Read the model definition and answer for the solid it produces. Units are mm, in the model's axes. Give positions to 0.01 mm unless a question says otherwise; leave off trailing zeros. Order: outer loops, then holes, each group sorted by start corner. A loop starts at its lowest first (then second) coordinate and runs counter-clockwise, first axis right, second up.
Item 1: A cutting plane is placed at B-B (z = 0.7). State how many separate pieces and enclosed holes the cut face has, plus the area to 3 significant figures.
Item 2: A cutting plane is placed at A-A (x = -188). Write down the section's boundary in (y, z), plus the area to 3 significant figures.
Item 3: Given pin 1 Ø3.5 at (x, y) = (-64.04, 35) entering from -Z; pin 2 Ø1.5 at (y, z) = (36.5, 2) entering from +X; pin 3 Ø0.9 at (x, z) = (-329, 1) entering from +Y; pin 4 Ø1.5 at (y, z) = (35, 2) entering from -X, each flat-ended and moving along its own axis, determine where each tip first touches the part or whether it passes through.
Item 4: A cutting plane is placed at C-C (x = -98). Write down the section's boundary in (y, z).
Item 5: Find the intervals of material crossed by line 1 along Y through (x, z) = (-47, 0.55); line 2 along X through (y, z) = (37, 1.1); line 3 along X through (y, z) = (54, 2.5), in increasing order.
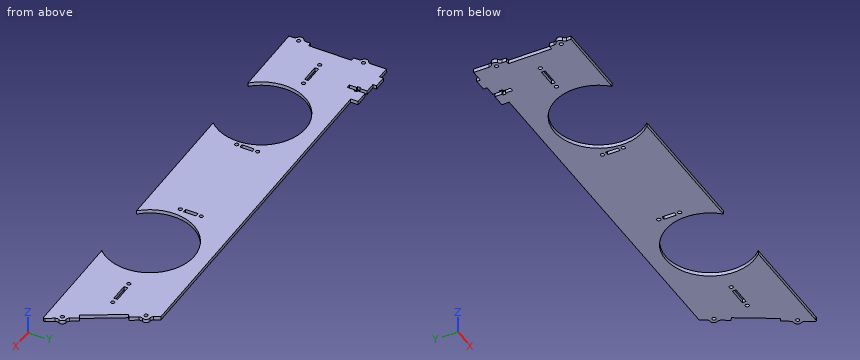
from build123d import *

# Parameters (mm, degrees)
EXTRUDE_1_DEPTH      = 3
SKETCH_2_W           = 3
SKETCH_2_H           = 35
CUT_EXTRUDE_1_DEPTH  = 3
CUT_EXTRUDE_2_DEPTH  = 3
SKETCH_4_W           = 3
SKETCH_4_H           = 10
CUT_EXTRUDE_3_DEPTH  = 3
SKETCH_5_W           = 15
SKETCH_5_H           = 3
CUT_EXTRUDE_4_DEPTH  = 3
SKETCH_6_W           = 42
SKETCH_6_H           = 3
EXTRUDE_2_DEPTH      = 6
SKETCH_8_W           = 3
SKETCH_8_H           = 3
SKETCH_9_W           = 3
SKETCH_9_H           = 3
SKETCH_7_R           = 1.5
CUT_EXTRUDE_6_DEPTH  = 3
FILLET_1_R           = 3
SKETCH_14_R          = 1.5
CUT_EXTRUDE_9_DEPTH  = 3
SKETCH_15_R          = 1.5
CUT_EXTRUDE_10_DEPTH = 3
SKETCH_16_W          = 3
SKETCH_16_H          = 3
SKETCH_17_W          = 3
SKETCH_17_H          = 3
SKETCH_18_R          = 1.5
CUT_EXTRUDE_11_DEPTH = 3
FILLET_2_R           = 3
SKETCH_19_R          = 36
CUT_EXTRUDE_12_DEPTH = 3
CUT_EXTRUDE_13_DEPTH = 3
SKETCH_21_W          = 10
SKETCH_21_H          = 3
EXTRUDE_3_DEPTH      = 3
FILLET_3_R           = 1


with BuildPart() as part:
    # Эскиз1 → Бобышка-Вытянуть1 (new body)
    with BuildSketch(Plane.XY):
        Polygon((-42.146569651, 73), (0, 0), (-366.876569651, 0), (-366.876569651, 73), align=None)
    extrude(amount=EXTRUDE_1_DEPTH)

    # Эскиз2 → Вырез-Вытянуть1 (cut)
    with BuildSketch(Plane.XY.offset(3)):
        with Locations((-365.376569651, 35)):
            Rectangle(SKETCH_2_W, SKETCH_2_H)
    extrude(amount=-CUT_EXTRUDE_1_DEPTH, mode=Mode.SUBTRACT)

    # Эскиз3 → Вырез-Вытянуть2 (cut)
    with BuildSketch(Plane.XY.offset(3)):
        Polygon((-33.287386441, 51.655444566), (-30.689310229, 53.155444566), (-13.189310229, 22.844555434), (-15.787386441, 21.344555434), align=None)
    extrude(amount=-CUT_EXTRUDE_2_DEPTH, mode=Mode.SUBTRACT)

    # Эскиз4 → Вырез-Вытянуть3 (cut)
    with BuildSketch(Plane.XY.offset(3)):
        with Locations((-240.376569651, 35)):
            Rectangle(SKETCH_4_W, SKETCH_4_H)
        with Locations((-156.376569651, 35)):
            Rectangle(SKETCH_4_W, SKETCH_4_H)
    extrude(amount=-CUT_EXTRUDE_3_DEPTH, mode=Mode.SUBTRACT)

    # Эскиз5 → Вырез-Вытянуть4 (cut)
    with BuildSketch(Plane.XY.offset(3)):
        with Locations((-336.376569651, 35)):
            Rectangle(SKETCH_5_W, SKETCH_5_H)
        with Locations((-52.036569651, 35)):
            Rectangle(SKETCH_5_W, SKETCH_5_H)
    extrude(amount=-CUT_EXTRUDE_4_DEPTH, mode=Mode.SUBTRACT)

    # Эскиз6 → Бобышка-Вытянуть2 (add)
    with BuildSketch(Plane(origin=(0, 73, 0), x_dir=(1, 0, 0), z_dir=(0, 1, 0))):
        with Locations((-345.876569651, -1.5)):
            Rectangle(SKETCH_6_W, SKETCH_6_H)
    extrude(amount=EXTRUDE_2_DEPTH)

    # Эскиз8 → Повернуть1 (revolve)
    with BuildSketch(Plane.ZY.offset(366.876569651)):
        with Locations((1.5, 7.25)):
            Rectangle(SKETCH_8_W, SKETCH_8_H)
    revolve(axis=Axis((-366.876569651, 8.75, 0), (0, 0, 1)))

    # Эскиз9 → Повернуть2 (revolve)
    with BuildSketch(Plane.ZY.offset(366.876569651)):
        with Locations((1.5, 59.75)):
            Rectangle(SKETCH_9_W, SKETCH_9_H)
    revolve(axis=Axis((-366.876569651, 61.25, 0), (0, 0, 1)))

    # Эскиз7 → Вырез-Вытянуть6 (cut)
    with BuildSketch(Plane.XY.offset(3)):
        with Locations((-365.376569651, 8.75)):
            Circle(SKETCH_7_R)
        with Locations(Location((-365.376569651, 61.25, 0), (0, 0, 180))):
            Circle(SKETCH_7_R)
    extrude(amount=-CUT_EXTRUDE_6_DEPTH, mode=Mode.SUBTRACT)

    # Скругление1
    fillet_1_edges = [part.edges().sort_by_distance(p)[0] for p in [
        (-366.876569651, 5.75, 1.5),
        (-366.876569651, 11.75, 1.5),
        (-366.876569651, 58.25, 1.5),
        (-366.876569651, 64.25, 1.5),
    ]]
    fillet(fillet_1_edges, radius=FILLET_1_R)

    # Эскиз14 → Вырез-Вытянуть9 (cut)
    with BuildSketch(Plane.XY.offset(3)):
        with Locations((-156.376569651, 43.5)):
            Circle(SKETCH_14_R)
        with Locations((-156.376569651, 26.5)):
            Circle(SKETCH_14_R)
        with Locations((-240.376569651, 26.5)):
            Circle(SKETCH_14_R)
        with Locations((-240.376569651, 43.5)):
            Circle(SKETCH_14_R)
    extrude(amount=-CUT_EXTRUDE_9_DEPTH, mode=Mode.SUBTRACT)

    # Эскиз15 → Вырез-Вытянуть10 (cut)
    with BuildSketch(Plane.XY.offset(3)):
        with Locations((-324.376569651, 35)):
            Circle(SKETCH_15_R)
        with Locations((-348.376569651, 35)):
            Circle(SKETCH_15_R)
        with Locations((-64.036569651, 35)):
            Circle(SKETCH_15_R)
        with Locations((-40.036569651, 35)):
            Circle(SKETCH_15_R)
    extrude(amount=-CUT_EXTRUDE_10_DEPTH, mode=Mode.SUBTRACT)

    # Эскиз16 → Повернуть3 (revolve)
    with BuildSketch(Plane(origin=(0, 0, 0), x_dir=(0, 0, -1), z_dir=(0.8660254037844265, 0.5000000000000212, 0))):
        with Locations((-1.5, 12.558620458)):
            Rectangle(SKETCH_16_W, SKETCH_16_H)
    revolve(axis=Axis((-7.029310229, 12.175122459, 3), (0, 0, -1)))

    # Эскиз17 → Повернуть4 (revolve)
    with BuildSketch(Plane(origin=(0, 0, 0), x_dir=(0, 0, -1), z_dir=(0.8660254037844265, 0.5000000000000212, 0))):
        with Locations((-1.5, 75.198620458)):
            Rectangle(SKETCH_17_W, SKETCH_17_H)
    revolve(axis=Axis((-36.849310229, 63.824877541, 3), (0, 0, -1)))

    # Эскиз18 → Вырез-Вытянуть11 (cut)
    with BuildSketch(Plane.XY.offset(3)):
        with Locations((-38.149990748, 63.077722283)):
            Circle(SKETCH_18_R)
        with Locations((-8.326705922, 11.422277717)):
            Circle(SKETCH_18_R)
    extrude(amount=-CUT_EXTRUDE_11_DEPTH, mode=Mode.SUBTRACT)

    # Скругление2
    fillet_2_edges = [part.edges().sort_by_distance(p)[0] for p in [
        (-5.529310229, 9.577046248, 1.5),
        (-8.529310229, 14.773198671, 1.5),
        (-35.349310229, 61.226801329, 1.5),
        (-38.349310229, 66.422953752, 1.5),
    ]]
    fillet(fillet_2_edges, radius=FILLET_2_R)

    # Эскиз19 → Вырез-Вытянуть12 (cut)
    with BuildSketch(Plane.XY.offset(3)):
        with Locations((-279.876569651, 25)):
            Circle(SKETCH_19_R)
        with Locations((-113.876569651, 25)):
            Circle(SKETCH_19_R)
    extrude(amount=-CUT_EXTRUDE_12_DEPTH, mode=Mode.SUBTRACT)

    # Эскиз20 → Вырез-Вытянуть13 (cut)
    with BuildSketch(Plane.XY.offset(3)):
        Polygon((-338.376569651, 79), (-338.376569651, 73), (-339.626569651, 73), (-339.626569651, 70.5), (-338.376569651, 70.5), (-338.376569651, 64.5), (-335.376569651, 64.5), (-335.376569651, 70.5), (-334.126569651, 70.5), (-334.126569651, 73), (-335.376569651, 73), (-335.376569651, 79), align=None)
    extrude(amount=-CUT_EXTRUDE_13_DEPTH, mode=Mode.SUBTRACT)

    # Эскиз21 → Бобышка-Вытянуть3 (add)
    with BuildSketch(Plane(origin=(0, 79, 0), x_dir=(1, 0, 0), z_dir=(0, 1, 0))):
        with Locations((-351.876569651, -1.5)):
            Rectangle(SKETCH_21_W, SKETCH_21_H)
    extrude(amount=EXTRUDE_3_DEPTH)

    # Скругление3
    fillet_3_edges = [part.edges().sort_by_distance(p)[0] for p in [
        (0, 0, 1.5),
    ]]
    fillet(fillet_3_edges, radius=FILLET_3_R)


solid = part.part
Response values:
1. separate pieces: 1
1. enclosed holes: 16
1. area: 17,700 mm2
2. outline: (0, 0) - (73, 0) - (73, 3) - (0, 3) - close
2. area: 219 mm2
3. pin 1: stops at z = 0
3. pin 2: stops at x = -24.1
3. pin 3: stops at y = 79
3. pin 4: stops at x = -363.88
4. outline: (57.31, 0) - (73, 0) - (73, 3) - (57.31, 3) - close
5. line 1: y = 0 to 33.5, 36.5 to 73
5. line 2: x = -363.88 to -313.82, -245.94 to -241.88, -238.88 to -157.88, -154.88 to -147.82, -79.94 to -24.83
5. line 3: x = -366.88 to -301.21, -258.55 to -135.21, -92.55 to -31.18
